The figure shows three views and two pictorial views of one solid part (mm, origin at its lowest corner). Answer the questions. Give positions to 0.01 mm unless a question says otherwise; leave off trailing zeros. Write each loop counter-clockwise with the first axis right and the second up, starting at its lowest first coordinate (ties: lowest second). Pieces come first, ordered by that corner, then holes. Notation, with made-up numbers: M -32,14.5 L 13,14.5 A16 cw 13,29.5 Z; hole C 58,-12 d8. An arc over 180 degrees is marked long. Return JSON: item names as keys, results as strings.
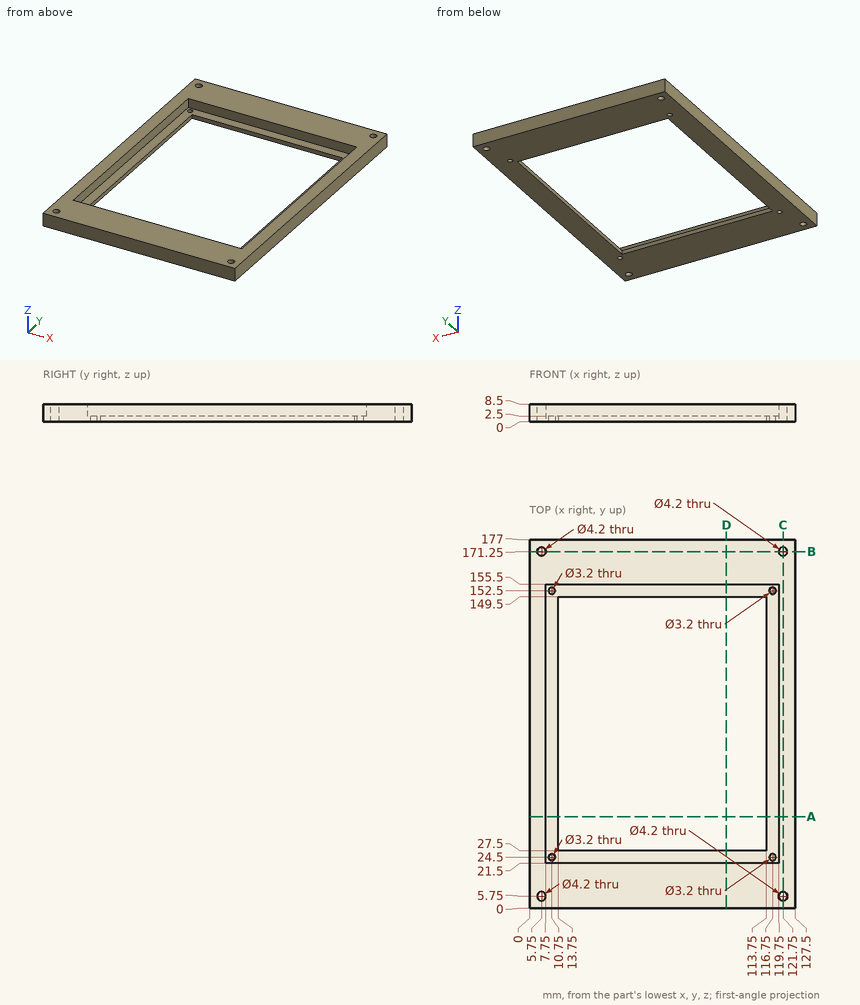
Item 1: A cutting plane is placed at A-A, the plane y = 44. Write down the section's boundary in (x, z), plus the area to 3 significant figures.
Geometry results:
{"outline": "M 0,0 L 13.75,0 L 13.75,2.5 L 7.75,2.5 L 7.75,8.5 L 0,8.5 Z; M 113.75,0 L 127.5,0 L 127.5,8.5 L 119.75,8.5 L 119.75,2.5 L 113.75,2.5 Z", "area": "162 mm2"}
Item 2: A cutting plane is placed at D-D, the plane x = 94.5. Write down the section's boundary in (y, z).
Geometry results:
{"outline": "M 0,0 L 27.5,0 L 27.5,2.5 L 21.5,2.5 L 21.5,8.5 L 0,8.5 Z; M 149.5,0 L 177,0 L 177,8.5 L 155.5,8.5 L 155.5,2.5 L 149.5,2.5 Z"}
Item 3: Given pin 1 Ø5 at (y, z) = (84.5, 3.5) entering from -X, flat-ended and moving along its own axis, determine where the tip first touches the part or whether it passes through.
Geometry results:
{"pin 1": "stops at x = 0"}
Item 4: Find the intervals of material crossed by line 1 (Y direction, x = 121.75, z = 3); line 2 (X direction, y = 152.5, z = 0.5); line 3 (X direction, y = 80, z = 3), in increasing order.
Geometry results:
{"line 1": "y = 0 to 3.65, 7.85 to 169.15, 173.35 to 177", "line 2": "x = 0 to 9.15, 12.35 to 115.15, 118.35 to 127.5", "line 3": "x = 0 to 7.75, 119.75 to 127.5"}
Item 5: A cutting plane is placed at B-B, the plane y = 171.25. Write down the section's boundary in (x, z), plus the area to 3 significant figures.
Geometry results:
{"outline": "M 0,0 L 3.65,0 L 3.65,8.5 L 0,8.5 Z; M 7.85,0 L 119.65,0 L 119.65,8.5 L 7.85,8.5 Z; M 123.85,0 L 127.5,0 L 127.5,8.5 L 123.85,8.5 Z", "area": "1,010 mm2"}
Item 6: A cutting plane is placed at C-C, the plane x = 121.75. Write down the section's boundary in (y, z), plus the area to 3 significant figures.
Geometry results:
{"outline": "M 0,0 L 3.65,0 L 3.65,8.5 L 0,8.5 Z; M 7.85,0 L 169.15,0 L 169.15,8.5 L 7.85,8.5 Z; M 173.35,0 L 177,0 L 177,8.5 L 173.35,8.5 Z", "area": "1,430 mm2"}
